Geometry: see drawing. Coordinates: mm, zero at the bounding-box minimum. A direction names the side the tool comes from. Give positions to 0.01 mm unless a question says otherwise; leave off trailing zeros. Write each loop counter-clockwise with the first axis right and the second up, starting at its lowest first coordinate (ties: lowest second). Pieces come first, ordered by that corner, then holes. Notation, with made-up numbers: M -15.5,86 L 3.5,86 A21 cw 3.5,115 Z; hole C 42,63 d8. An arc over 180 degrees is marked long. Use one line per item in the form item = value. Start each with the question number.
Item 1: Contact query for flat-ended pins moving along their axis: P1, Ø1.5, axis at x = 26, z = 77.5, coming from the +Y side; P2, Ø10, axis at x = 121, y = 177, coming from the -Z side; P3, Ø5, axis at x = 48, z = 88.5, coming from the -Y side. Output: stop coordinate, or through.
Item 2: Section query C-C on y = 923. Return loops of the section in (x, z), then the cut area to 3 significant figures.
Item 3: Section query D-D on z = 144. Return loops of the section in (x, y).
Item 4: Access query for the marked faces 1, 2 and 3. Directions: +Z, -Z, +X, -X, +Y, -Y. A direction counts if a zero-diameter tool reaches every point of the face in a straight line with its end or side. Return the directions, or none.
Item 5: Material intervals for line 1 along Y through (x, z) = (68, 26); line 2 along X through (y, z) = (1159, 77.5); line 3 along X through (y, z) = (1119.5, 86), sorted ascending. Write a range as from..to.
Item 6: Section query A-A on z = 80. Return loops of the section in (x, y), then the cut area to 3 significant figures.
Item 7: Section query B-B on x = 80. Return loops of the section in (y, z).
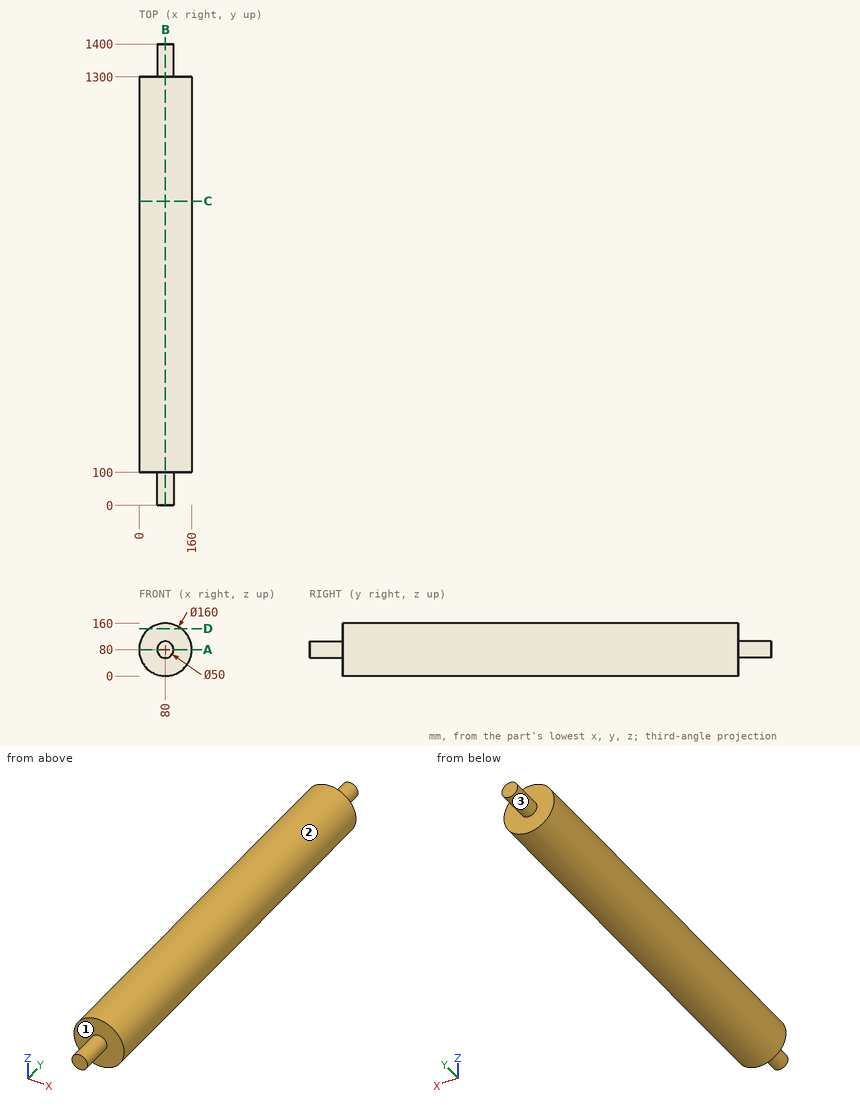
Answer sheet:
q1.P1 = 1300
q1.P2 = 8.56
q1.P3 = 100
q2.outline = C 80,80 d160
q2.area = 20,100 mm2
q3.outline = M 32,100 L 128,100 L 128,1300 L 32,1300 Z
q4.face_1 = -Y
q4.face_2 = +Y, -Y
q4.face_3 = +Y
q5.line_1 = 100..1300
q5.line_2 = 0.04..159.96
q5.line_3 = 0.23..159.77
q6.outline = M 0,100 L 55,100 L 55,0 L 105,0 L 105,100 L 160,100 L 160,1300 L 105,1300 L 105,1400 L 55,1400 L 55,1300 L 0,1300 Z
q6.area = 202,000 mm2
q7.outline = M 0,55 L 100,55 L 100,0 L 1300,0 L 1300,55 L 1400,55 L 1400,105 L 1300,105 L 1300,160 L 100,160 L 100,105 L 0,105 Z
